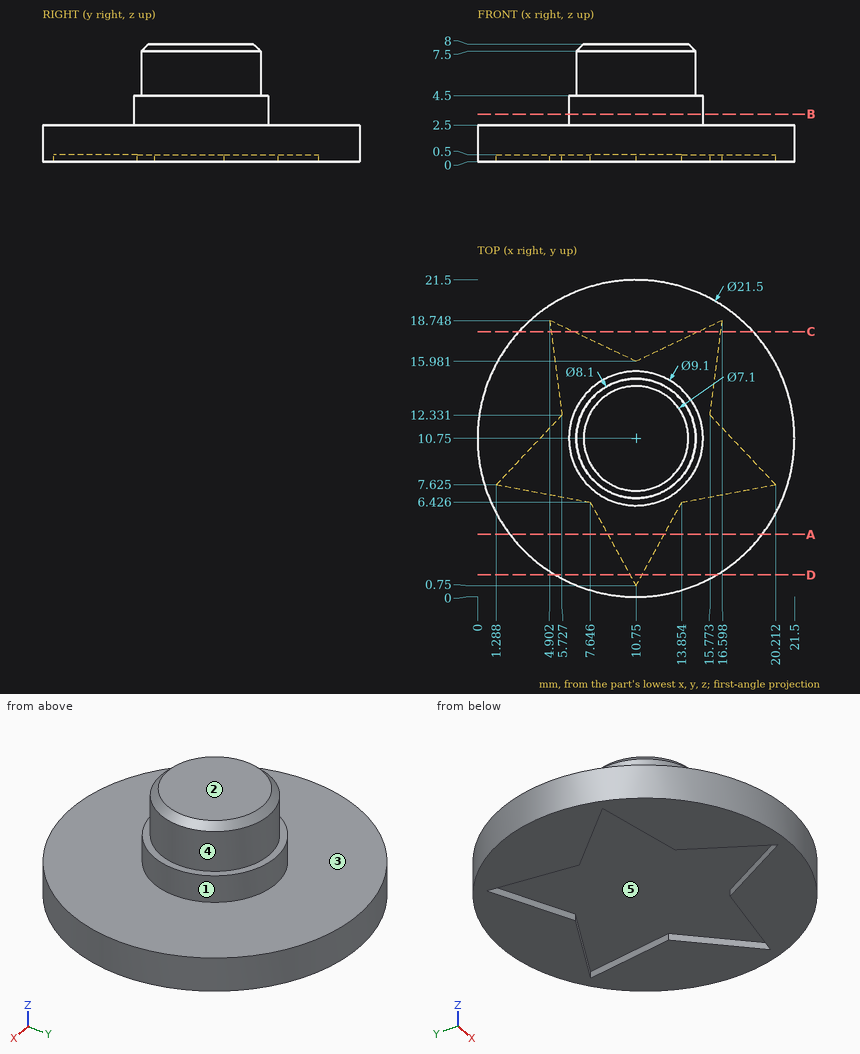
Could you check a few things on this drawing? It's one solid part, dimensions in mm from its lowest x, y, z. A direction names the side the tool comes from. Coordinates: 2 decimals unless noted, no trailing zeros. Order: outer loops, then holes, each group sorted by start corner. A loop starts at its lowest first (then second) coordinate and runs counter-clockwise, first axis right, second up.
1) Will this pin go through, and if not, where does the flat tip stop? pin 1 (2 mm diameter, centred on x = 6, z = 5.5, fed in from -Y).
2) Imagine slicing it at D-D on y = 1.5. List the corners of the cut face in (x, z) for me.
3) Imagine slicing it at C-C on y = 18. List the corners of the cut face in (x, z) for me, and give its area (3 significant figures).
4) Imagine slicing it at B-B on z = 3.25. List the corners of the cut face in (x, y) for me.
5) I need wall thicknesses on line 1 (Z direction, x = 17.5, y = 16.75); line 2 (Z direction, x = 3.5, y = 7.75); line 3 (Y direction, x = 9.25, z = 4) (1 decimal). Which ranges of each line are inside material? Lowest first, please.
6) Imagine slicing it at A-A on y = 4.25. List the corners of the cut face in (x, z) for me (1 decimal).
7) Which directions (+Z, -Z, +X, -X, +Y, -Y) give clear straight access to the entire face, cutting with the end or side of a thin tool? Please do the marked faces 1 and 2.
8) We'd pull the mould along X, two halves only. Please class the marked faces 3, 4 and 5: +X half, -X half, draft (parallel to the pull), parting line (faces both ways), or undercut.
Response values:
1. pin 1: stops at y = 9.22
2. outline: (5.27, 0) - (10.34, 0) - (10.34, 0.5) - (11.16, 0.5) - (11.16, 0) - (16.23, 0) - (16.23, 2.5) - (5.27, 2.5) - close
3. outline: (2.81, 0) - (5, 0) - (5, 0.5) - (6.48, 0.5) - (6.48, 0) - (15.02, 0) - (15.02, 0.5) - (16.5, 0.5) - (16.5, 0) - (18.69, 0) - (18.69, 2.5) - (2.81, 2.5) - close
3. area: 38.2 mm2
4. outline: circle Ø9.1 at (10.75, 10.75)
5. line 1: z = 0 to 2.5
5. line 2: z = 0.5 to 2.5
5. line 3: y = 6.5 to 15
6. outline: (2.2, 0) - (8.8, 0) - (8.8, 0.5) - (12.7, 0.5) - (12.7, 0) - (19.3, 0) - (19.3, 2.5) - (2.2, 2.5) - close
7. face 1: +Z
7. face 2: +Z, +X, -X, +Y, -Y
8. face 3: draft
8. face 4: parting line
8. face 5: undercut
